The listing builds one solid part. Answer for the finished solid, in the listing's coordinates (mm). Face numbers are marked on the shaded views. A direction names the side the tool comes from. Give positions to 0.01 mm unless a question says otherwise; leave off trailing zeros. Loops run counter-clockwise (first coordinate to the right, second up) from the corner with the lowest first, then second, coordinate; pieces in that order, holes last.
Item 1: Section A-A, the plane z = 1 is taken. Give the vertices of the cut face in (x, y).
Item 2: A tool of negligible diameter and unlimited length cuts with its end or side. For the marked faces 4, 5 and 6, from which of +Z, -Z, +X, -X, +Y, -Y can it reach the whole face along a straight path? Write none if from no direction.
Item 3: Section D-D, the plane y = 6.35 is taken. Give the vertices of the cut face in (x, z), and give its area (3 significant figures).
Item 4: Section C-C, the plane x = 0.25 is taken. Give the vertices of the cut face in (y, z), and give its area (3 significant figures).
Item 5: Consider line 1 along Y through (x, z) = (0, 0.45); line 2 along X through (y, z) = (0, 1.1); line 3 along X through (y, z) = (3.25, 0.3). Determine where each line is inside the solid, lowest interval first.
Item 6: Each of these flat-tipped pins is pushed along its axis until it touches: pin 1 Ø1.4 at (x, y) = (0, 0.5) entering from +Z; pin 2 Ø1.5 at (x, y) = (-1, -3) entering from +Z; pin 3 Ø0.5 at (y, z) = (-2.5, 1.5) entering from +X. Where does it stop, or does it pass through?
Item 7: The mould has two halves that part along Y. Classify the marked faces 1, 2 and 3: pulls with the +Y half, pulls with the -Y half, needs draft (parallel to the pull), parting line crosses it, or undercut.
Item 8: Section B-B, the plane y = 0 is taken. Give the vertices of the cut face in (x, z), and give its area (3 significant figures).
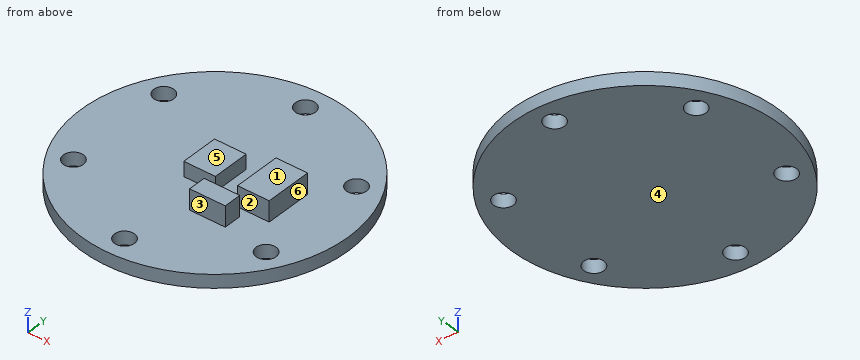
from build123d import *

# Parameters (mm, degrees)
F0_R     = 7.62
F1_DEPTH = 0.762
F2_R     = 0.5715
F3_DEPTH = 0.762
F4_W     = 1.8034
F4_H     = 2.159
F5_DEPTH = 1.6002
F6_W     = 2.032
F6_H     = 1.016
F6_W_2   = 1.8034
F6_H_2   = 2.6924
F7_DEPTH = 1.9304


with BuildPart() as f1:
    # F0 (on Top) → F1 (new body)
    with BuildSketch(Plane.XY):
        Circle(F0_R)
    extrude(amount=F1_DEPTH)

    # F2 (on face) → F3 (cut, through all)
    with BuildSketch(Plane.XY.offset(0.762)):
        with Locations((0, 6.35)):
            Circle(F2_R)
        with Locations((-5.499261, 3.175)):
            Circle(F2_R)
        with Locations((-5.499261, -3.175)):
            Circle(F2_R)
        with Locations((0, -6.35)):
            Circle(F2_R)
        with Locations((5.499261, -3.175)):
            Circle(F2_R)
        with Locations((5.499261, 3.175)):
            Circle(F2_R)
    extrude(amount=-F3_DEPTH, mode=Mode.SUBTRACT)

    # F4 (on face) → F5 (join)
    with BuildSketch(Plane(origin=(0, 0, 0), x_dir=(1, 0, 0), z_dir=(0, 0, -1))):
        Rectangle(F4_W, F4_H)
    extrude(amount=-F5_DEPTH)

    # F6 (on face) → F7 (join)
    with BuildSketch(Plane(origin=(0, 0, 0), x_dir=(1, 0, 0), z_dir=(0, 0, -1))):
        with Locations((1.905, 2.3622)):
            Rectangle(F6_W, F6_H)
        with Locations((3.2893, 0)):
            Rectangle(F6_W_2, F6_H_2)
    extrude(amount=-F7_DEPTH)


solid = f1.part
Worked answers:
1. outline: (-0.9, -1.08) - (0.9, -1.08) - (0.9, 1.08) - (-0.9, 1.08) - close; (0.89, -2.87) - (2.92, -2.87) - (2.92, -1.85) - (0.89, -1.85) - close; (2.39, -1.35) - (4.19, -1.35) - (4.19, 1.35) - (2.39, 1.35) - close
2. face 4: -Z, +X, -X, +Y, -Y
2. face 5: +Z, -X, +Y, -Y
2. face 6: +Z, +X, +Y, -Y
3. outline: (-4.21, 0) - (-0.57, 0) - (-0.57, 0.76) - (-4.21, 0.76) - close; (0.57, 0) - (4.21, 0) - (4.21, 0.76) - (0.57, 0.76) - close
3. area: 5.55 mm2
4. outline: (-7.62, 0) - (-6.86, 0) - (-6.86, 0.76) - (-7.62, 0.76) - close; (-5.84, 0) - (5.84, 0) - (5.84, 0.76) - (1.08, 0.76) - (1.08, 1.6) - (-1.08, 1.6) - (-1.08, 0.76) - (-5.84, 0.76) - close; (6.86, 0) - (7.62, 0) - (7.62, 0.76) - (6.86, 0.76) - close
4. area: 11.8 mm2
5. line 1: y = -7.62 to -6.92, -5.78 to 5.78, 6.92 to 7.62
5. line 2: x = -0.9 to 0.9, 2.39 to 4.19
5. line 3: x = -6.89 to -6.07, -4.93 to 4.93, 6.07 to 6.89
6. pin 1: stops at z = 1.6
6. pin 2: stops at z = 0.76
6. pin 3: stops at x = 2.92
7. face 1: needs draft
7. face 2: undercut
7. face 3: pulls with the -Y half
8. outline: (-7.62, 0) - (7.62, 0) - (7.62, 0.76) - (4.19, 0.76) - (4.19, 1.93) - (2.39, 1.93) - (2.39, 0.76) - (0.9, 0.76) - (0.9, 1.6) - (-0.9, 1.6) - (-0.9, 0.76) - (-7.62, 0.76) - close
8. area: 15.2 mm2
